Autodesk Inventor part; units mm, degrees
ref_plane "YZ Plane" through (0, 0, 0) normal (1, 0, 0) x (0, 1, 0)
ref_plane "XZ Plane" through (0, 0, 0) normal (0, 1, 0) x (-1, 0, 0)
ref_plane "XY Plane" through (0, 0, 0) normal (0, 0, 1) x (1, 0, 0)
sketch "Sketch1" plane through (0, 0, 0) normal (0, 0, 1) x (1, 0, 0)
  line L0 (-2.5, 0) -> (-2.5, 8)
  line L1 (-2.5, 8) -> (-1.7679, 8)
  line L2 (-1.7679, 8) -> (-1.5, 7)
  line L3 (-1.5, 7) -> (0, 7)
  line L4 (0, 0) -> (0, 14.5205) construction
  line L5 (-2.5, 0) -> (2.5, 0)
  line L6 (2.5, 0) -> (2.5, 8)
  line L7 (2.5, 8) -> (1.7679, 8)
  line L8 (1.7679, 8) -> (1.5, 7)
  line L9 (1.5, 7) -> (0, 7)
  dimension "d0" = 5
  dimension "d1" = 16
  dimension "d2" = 14
  dimension "d3" = 3
  dimension "d4" = 15
revolve "Revolution1" add sketch "Sketch1" angle 360 about axis through (-2.5, 0, 0) along (1, 0, 0)
sketch "Sketch2" plane through (0, 0, 0) normal (0, 0, 1) x (1, 0, 0)
  circle A0 centre (0, 0) radius 0.75
  dimension "d6" = 1.5
extrude "Extrusion1" cut sketch "Sketch2" along normal blind 10 and the other way blind 10
sketch "Sketch4" plane through (-2.5, 0, 0) normal (-1, 0, 0) x (0, 0, 1)
  circle A0 centre (0, 0) radius 2
  dimension "d18" = 4
extrude "Extrusion2" cut sketch "Sketch4" against normal through all
sketch "Sketch7" plane through (0, 0, 0) normal (0, 0, 1) x (1, 0, 0)
  circle A0 centre (0, 4.5) radius 1
  point P0 (0, 0)
  dimension "d32" = 2
  dimension "d33" = 4.5
extrude "Extrusion3" cut sketch "Sketch7" along normal through all both and the other way through all
properties part number "spool v2"
Here's how the part is built. I have some questions about the finished solid (model axes, mm). A direction names the side the tool comes from. Give positions to 0.01 mm unless a question says otherwise; leave off trailing zeros. Loops run counter-clockwise (first coordinate to the right, second up) from the corner with the lowest first, then second, coordinate; pieces in that order, holes last. Notation, with made-up numbers: (41.5, 55.5) -> (46.5, 55.5) arc R20 cw to (46.5, 80.5) -> close; hole circle Ø8 at (20.5, 64.25). An arc over 180 degrees is marked (long way). Use one line per item in the form item = value. Start each with the question number.
1) Thinking about a two-plate mould opening in Z: for faces 3 (the face through (-0.035, -1.774, 0.923)), 4 (the face through (-2.5, 2, -2)), 5 (the face through (2.13, -1.73, 7.81)), which applies, +Z half, -Z half, draft (parallel to the pull), parting line (faces both ways), or undercut?
2) Imagine slicing it at C-C (x = 0). Please give me the cut outline in (y, z), then the cut area to 3 significant figures.
3) Imagine slicing it at D-D (x = -2). Please give me the cut outline in (y, z).
4) Imagine slicing it at B-B (y = 0). Please give me the cut outline in (x, z).
5) Which directions (+Z, -Z, +X, -X, +Y, -Y) give clear straight access to the entire face, cutting with the end or side of a thin tool? Please do faces 1 (the face through (0.021, -1.517, -6.834)), 2 (the face through (-0.217, 3.524, 0.085)).
6) Imagine slicing it at A-A (z = 0). Please give me the cut outline in (x, y), then the cut area to 3 significant figures.
7) For P1, Ø1.7, axis at x = 0, y = 0, coming from the +Z side; P2, Ø1.5, axis at x = -1.5, y = -3, coming from the +Z side, each with a flat end and sliding along its axis, tell me the tip position at first contact or that it passes through.
8) Please list where these lines run through material, in increasing order: line 1 along X through (y, z) = (4.5, 0.75); line 2 along Z through (x, y) = (0.8, 0); line 3 along X through (y, z) = (0, 5.75).
Check values:
q1.face_3 = undercut
q1.face_4 = draft
q1.face_5 = parting line
q2.outline = (-0.75, -6.96) -> (-0.75, -1.85) arc R2 cw to (-0.75, 1.85) -> (-0.75, 6.96) arc R7 ccw to start; (0.75, -6.96) arc R7 ccw to (3.5, -6.06) -> (3.5, 6.06) arc R7 ccw to (0.75, 6.96) -> (0.75, 1.85) arc R2 cw to (0.75, -1.85) -> close; (5.5, -4.33) arc R7 ccw to (5.5, 4.33) -> close
q2.area = 105 mm^2
q3.outline = circle Ø16 at (0, 0); hole circle Ø4 at (0, 0)
q4.outline = (-2.5, -8) -> (-1.77, -8) -> (-1.5, -7) -> (-0.75, -7) -> (-0.75, -2) -> (-2.5, -2) -> close; (-2.5, 2) -> (-0.75, 2) -> (-0.75, 7) -> (-1.5, 7) -> (-1.77, 8) -> (-2.5, 8) -> close; (0.75, -7) -> (1.5, -7) -> (1.77, -8) -> (2.5, -8) -> (2.5, -2) -> (0.75, -2) -> close; (0.75, 2) -> (2.5, 2) -> (2.5, 8) -> (1.77, 8) -> (1.5, 7) -> (0.75, 7) -> close
q5.face_1 = none
q5.face_2 = +Z, -Z
q6.outline = (-2.5, -8) -> (-1.77, -8) -> (-1.5, -7) -> (1.5, -7) -> (1.77, -8) -> (2.5, -8) -> (2.5, -2) -> (-2.5, -2) -> close; (-2.5, 2) -> (2.5, 2) -> (2.5, 8) -> (1.77, 8) -> (1.5, 7) -> (-1.5, 7) -> (-1.77, 8) -> (-2.5, 8) -> close; hole circle Ø2 at (0, 4.5)
q6.area = 50.3 mm^2
q7.P1 = 7
q7.P2 = 7.66
q8.line_1 = -2.5 to -1, 1 to 2.5
q8.line_2 = -7 to -2, 2 to 7
q8.line_3 = -2.5 to -0.75, 0.75 to 2.5
